from build123d import *

# Parameters (mm, degrees)
SKETCH1_W             = 45
SKETCH1_H             = 17.78
BOSS_EXTRUDE1_DEPTH   = 14
SKETCH1_W_2           = 15.24
SKETCH1_H_2           = 20.32
BOSS_EXTRUDE1_2_DEPTH = 14
BOSS_EXTRUDE1_3_DEPTH = 14
SKETCH1_W_3           = 18
SKETCH1_H_3           = 18
BOSS_EXTRUDE1_4_DEPTH = 14
SKETCH2_W             = 12.5
SKETCH2_H             = 5.7
BOSS_EXTRUDE2_DEPTH   = 7
BOSS_EXTRUDE2_2_DEPTH = 7
SKETCH2_W_2           = 7.5
BOSS_EXTRUDE2_3_DEPTH = 7
SKETCH4_W             = 9
SKETCH4_H             = 27.5
BOSS_EXTRUDE4_DEPTH   = 5
SKETCH5_W             = 7.5
SKETCH5_H             = 10
BOSS_EXTRUDE5_DEPTH   = 10
SKETCH3_W             = 57
SKETCH3_H             = 46.8
SKETCH3_R             = 1.6
BOSS_EXTRUDE3_DEPTH   = 1.5
SKETCH6_W             = 9.2
SKETCH6_H             = 7.6
BOSS_EXTRUDE6_DEPTH   = 4
FILLET1_R             = 2


with BuildPart() as part:
    # Sketch1 → Boss-Extrude1 (new body)
    with BuildSketch(Plane(origin=(0, 0, 0), x_dir=(1, 0, 0), z_dir=(0, 1, 0))):
        with Locations((22.5, 8.89)):
            Rectangle(SKETCH1_W, SKETCH1_H)
    extrude(amount=BOSS_EXTRUDE1_DEPTH)



with BuildPart() as body_2:
    # Sketch1 → Boss-Extrude1 2 (new body)
    with BuildSketch(Plane(origin=(0, 0, 0), x_dir=(1, 0, 0), z_dir=(0, 1, 0))):
        with Locations((30.88, -12.66)):
            Rectangle(SKETCH1_W_2, SKETCH1_H_2)
    extrude(amount=BOSS_EXTRUDE1_2_DEPTH)


with BuildPart() as body_3:
    # Sketch1 → Boss-Extrude1 3 (new body)
    with BuildSketch(Plane(origin=(0, 0, 0), x_dir=(1, 0, 0), z_dir=(0, 1, 0))):
        with Locations((13.94, -12.66)):
            Rectangle(SKETCH1_W_2, SKETCH1_H_2)
    extrude(amount=BOSS_EXTRUDE1_3_DEPTH)


with BuildPart() as body_4:
    # Sketch1 → Boss-Extrude1 4 (new body)
    with BuildSketch(Plane(origin=(0, 0, 0), x_dir=(1, 0, 0), z_dir=(0, 1, 0))):
        with Locations((-5.38, -11.5)):
            Rectangle(SKETCH1_W_3, SKETCH1_H_3)
    extrude(amount=BOSS_EXTRUDE1_4_DEPTH)


with BuildPart() as body_5:
    # Sketch2 → Boss-Extrude2 (new body)
    with BuildSketch(Plane(origin=(0, 0, 0), x_dir=(1, 0, 0), z_dir=(0, 1, 0))):
        with Locations((32.25, -26.17)):
            Rectangle(SKETCH2_W, SKETCH2_H)
    extrude(amount=BOSS_EXTRUDE2_DEPTH)


with BuildPart() as body_6:
    # Sketch2 → Boss-Extrude2 2 (new body)
    with BuildSketch(Plane(origin=(0, 0, 0), x_dir=(1, 0, 0), z_dir=(0, 1, 0))):
        with Locations((19.25, -26.17)):
            Rectangle(SKETCH2_W, SKETCH2_H)
    extrude(amount=BOSS_EXTRUDE2_2_DEPTH)


with BuildPart() as body_7:
    # Sketch2 → Boss-Extrude2 3 (new body)
    with BuildSketch(Plane(origin=(0, 0, 0), x_dir=(1, 0, 0), z_dir=(0, 1, 0))):
        with Locations((-0.13, -26.17)):
            Rectangle(SKETCH2_W_2, SKETCH2_H)
    extrude(amount=BOSS_EXTRUDE2_3_DEPTH)


with BuildPart() as body_8:
    # Sketch4 → Boss-Extrude4 (new body)
    with BuildSketch(Plane(origin=(0, 0, 0), x_dir=(1, 0, 0), z_dir=(0, 1, 0))):
        with Locations((-7.5, -6.75)):
            Rectangle(SKETCH4_W, SKETCH4_H)
    extrude(amount=BOSS_EXTRUDE4_DEPTH)


with BuildPart() as body_9:
    # Sketch5 → Boss-Extrude5 (new body)
    with BuildSketch(Plane(origin=(0, 0, 0), x_dir=(1, 0, 0), z_dir=(0, 1, 0))):
        with Locations((-4.75, 12.78)):
            Rectangle(SKETCH5_W, SKETCH5_H)
    extrude(amount=BOSS_EXTRUDE5_DEPTH)


with BuildPart() as part_1:
    add(part.part)

    add(body_2.part)  # Boss-Extrude3 merges body 2

    add(body_3.part)  # Boss-Extrude3 merges body 3

    add(body_4.part)  # Boss-Extrude3 merges body 4

    add(body_5.part)  # Boss-Extrude3 merges body 5

    add(body_6.part)  # Boss-Extrude3 merges body 6

    add(body_7.part)  # Boss-Extrude3 merges body 7

    add(body_8.part)  # Boss-Extrude3 merges body 8

    add(body_9.part)  # Boss-Extrude3 merges body 9
    # Sketch3 → Boss-Extrude3 (add)
    with BuildSketch(Plane(origin=(0, 0, 0), x_dir=(1, 0, 0), z_dir=(0, 1, 0))):
        with Locations((16.5, -5.62)):
            Rectangle(SKETCH3_W, SKETCH3_H)
        with Locations((41.5, -24.02)):
            Circle(SKETCH3_R, mode=Mode.SUBTRACT)
        with Locations((41.5, 8.48)):
            Circle(SKETCH3_R, mode=Mode.SUBTRACT)
        with Locations((18.5, 8.48)):
            Circle(SKETCH3_R, mode=Mode.SUBTRACT)
    extrude(amount=-BOSS_EXTRUDE3_DEPTH)

    # Sketch6 → Boss-Extrude6 (add)
    with BuildSketch(Plane(origin=(0, 14, 0), x_dir=(1, 0, 0), z_dir=(0, 1, 0))):
        with Locations((40.4, 8.89)):
            Rectangle(SKETCH6_W, SKETCH6_H)
    extrude(amount=BOSS_EXTRUDE6_DEPTH)

    # Fillet1
    fillet1_edges = [part_1.edges().sort_by_distance(p)[0] for p in [
        (45, -0.75, 29.02),
        (-12, -0.75, 29.02),
        (-12, -0.75, -17.78),
    ]]
    fillet(fillet1_edges, radius=FILLET1_R)


solid = part_1.part
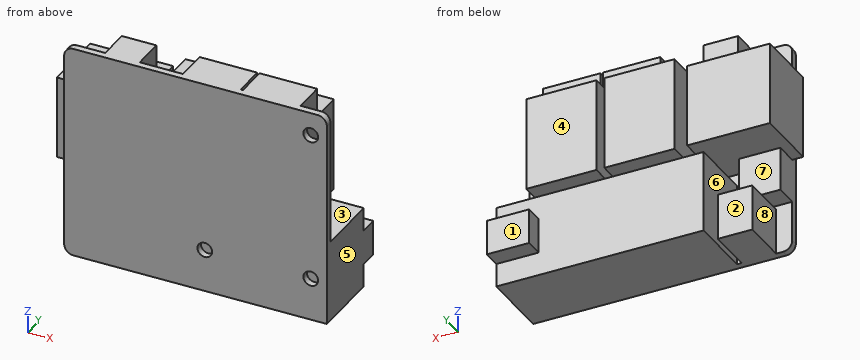
The model under review builds one solid part; all positions refer to its coordinate system, in mm. Face numbers are marked on the shaded views. A direction names the side the tool comes from. Round coordinates to 2 decimals unless told otherwise and drop trailing zeros. Loops run counter-clockwise (first coordinate to the right, second up) from the corner with the lowest first, then second, coordinate; pieces in that order, holes last. Notation, with made-up numbers: M 81,60 L 130,60 A21 ccw 130,76 Z; hole C 16,12.25 d3. An arc over 180 degrees is marked long. Answer as CSV lines item,"result".
1. We need section D-D (z = -8.48). Give the boundary of the cut face in (x, y).
Outcome:
outline,"M -12,-1.5 L 16.9,-1.5 L 16.9,0 L 20.1,0 L 20.1,-1.5 L 39.9,-1.5 L 39.9,0 L 43.1,0 L 43.1,-1.5 L 45,-1.5 L 45,18 L 35.8,18 L 35.8,14 L 0,14 L 0,0 L -1,0 L -1,10 L -8.5,10 L -8.5,0 L -12,0 Z"
2. Insertion check: pin 1 Ø4.5 at (x, z) = (32.5, 8.5) entering from +Y; pin 2 Ø1 at (x, z) = (19, -8.5) entering from -Y; pin 3 Ø1.7 at (y, z) = (2, 27) entering from +X. Each pin has a flat end and moves straight along its axis. Give the tip position at first contact, or say it passes through.
Outcome:
pin 1,"stops at y = 14"
pin 2,"stops at y = 0"
pin 3,"stops at x = 38.5"
3. We need section B-B (z = 24.02). Give the boundary of the cut face in (x, y).
Outcome:
outline,"M -12,-1.5 L 39.9,-1.5 L 39.9,0 L 38.5,0 L 38.5,7 L 26,7 L 26,0 L 25.5,0 L 25.5,7 L 13,7 L 13,0 L 3.62,0 L 3.62,7 L -3.88,7 L -3.88,0 L -12,0 Z; M 43.1,-1.5 L 45,-1.5 L 45,0 L 43.1,0 Z"
4. For the marked faces 1, 2, 3 and 4, list the 3-axis set-ups (+Z, -Z, +X, -X, +Y, -Y) from which the entire face can be reached by the end or side of a thin tool; tool diameter is ignored.
Outcome:
face 1,"+Z, -Z, +X, -X, +Y"
face 2,"-Z, -X, +Y"
face 3,"+X, +Y"
face 4,"+Z, +X, -X, +Y"
5. Draft analysis for pull direction X (two halves, no side actions). For the marked faces 5, 6, 7 and 8, state which applies: pulls with the +X half, pulls with the -X half, needs draft (parallel to the pull), parting line crosses it, or undercut.
Outcome:
face 5,"pulls with the +X half"
face 6,"undercut"
face 7,"needs draft"
face 8,"pulls with the -X half"
6. We need section A-A (x = 41.5). Give the boundary of the cut face in (y, z).
Outcome:
outline,"M -1.5,-17.78 L 14,-17.78 L 14,-12.69 L 18,-12.69 L 18,-5.09 L 14,-5.09 L 14,0 L 0,0 L 0,22.42 L -1.5,22.42 L -1.5,-6.88 L 0,-6.88 L 0,-10.08 L -1.5,-10.08 Z; M -1.5,25.62 L 0,25.62 L 0,29.02 L -1.5,29.02 Z"
7. To check wall thickness, follow L1, parallel to X at y = 3.5, z = 27.5; L2, parallel to Z at x = 41.5, y = -1.1; L3, parallel to X at y = -0.95, z = -8.48. State the ranges of each line that lie inside material, in increasing order. Write a range as [from, to].
Outcome:
L1,"x = [-3.88, 3.62], [13, 25.5], [26, 38.5]"
L2,"z = [-17.78, -10.08], [-6.88, 22.42], [25.62, 29.02]"
L3,"x = [-12, 16.9], [20.1, 39.9], [43.1, 45]"
8. We need section C-C (y = 11.5). Give the boundary of the cut face in (x, z), plus the area to 3 significant figures.
Outcome:
outline,"M -14.38,2.5 L 3.62,2.5 L 3.62,20.5 L -14.38,20.5 Z; M 0,-17.78 L 45,-17.78 L 45,0 L 0,0 Z; M 6.32,2.5 L 21.56,2.5 L 21.56,22.82 L 6.32,22.82 Z; M 23.26,2.5 L 38.5,2.5 L 38.5,22.82 L 23.26,22.82 Z"
area,"1,740 mm2"
